Check sheet for the modelled part. Datum: model origin and axes. Units: mm. A direction names the side the tool comes from. Give positions to 0.01 mm unless a question says otherwise; leave off trailing zeros. Order: outer loops, then holes, each group sorted by start corner. A loop starts at its lowest first (then second) coordinate and runs counter-clockwise, first axis right, second up.
from build123d import *

# Parameters (mm, degrees)
SKETCH1_W           = 12.7
SKETCH1_H           = 5.08
BOSS_EXTRUDE1_DEPTH = 63.5
SKETCH2_W           = 5.334
SKETCH2_H           = 30.734
CUT_EXTRUDE1_DEPTH  = 3.175


with BuildPart() as part:
    # Sketch1 → Boss-Extrude1 (new body)
    with BuildSketch(Plane.XY):
        Rectangle(SKETCH1_W, SKETCH1_H)
        with BuildLine():
            Line((-73.690101608, 45.085), (-78.089510659, 42.545))
            ThreePointArc((-78.089510659, 42.545), (0, -2.54), (78.089510659, 42.545))
            Line((78.089510659, 42.545), (73.690101608, 45.085))
            ThreePointArc((73.690101608, 45.085), (0, 2.54), (-73.690101608, 45.085))
        make_face()
    extrude(amount=BOSS_EXTRUDE1_DEPTH)

    # Sketch2 → Cut-Extrude1 (cut)
    with BuildSketch(Plane.XZ.offset(2.54)):
        with Locations((0.1143, 40.64)):
            Rectangle(SKETCH2_W, SKETCH2_H)
    extrude(amount=-CUT_EXTRUDE1_DEPTH, mode=Mode.SUBTRACT)


solid = part.part
1) Section check B-B, the plane z = 29. Record the cut outline in (x, y) (3 decimals).
Recorded:
outline: (-78.09, 42.545) arc R90.17 ccw to (-6.35, -2.316) - (-6.35, -2.54) - (-2.553, -2.54) - (-2.553, 0.635) - (2.781, 0.635) - (2.781, -2.54) - (6.35, -2.54) - (6.35, -2.316) arc R90.17 ccw to (78.09, 42.545) - (73.69, 45.085) arc R85.09 cw to (-73.69, 45.085) - close
2) Section check D-D, the plane z = 17.5. Record the cut outline in (x, y) (3 decimals).
Recorded:
outline: (-78.09, 42.545) arc R90.17 ccw to (-6.35, -2.316) - (-6.35, -2.54) - (6.35, -2.54) - (6.35, -2.316) arc R90.17 ccw to (78.09, 42.545) - (73.69, 45.085) arc R85.09 cw to (-73.69, 45.085) - close
3) Section check C-C, the plane y = 31.5. Record the cut outline in (x, z).
Recorded:
outline: (-70.57, 0) - (-63.95, 0) - (-63.95, 63.5) - (-70.57, 63.5) - close; (63.95, 0) - (70.57, 0) - (70.57, 63.5) - (63.95, 63.5) - close
4) Section check A-A, the plane y = 40.5. Record the cut outline in (x, z).
Recorded:
outline: (-76.87, 0) - (-70.85, 0) - (-70.85, 63.5) - (-76.87, 63.5) - close; (70.85, 0) - (76.87, 0) - (76.87, 63.5) - (70.85, 63.5) - close
5) Depth check by flat-ended pin: pin 1 Ø4 at (x, z) = (29.5, 34) entering from +Y; pin 2 Ø1.5 at (y, z) = (24.5, 41.5) entering from +X; pin 3 Ø3 at (y, z) = (9, 52) entering from +X. Enter the tip coordinate at first touch or a pass-through.
Recorded:
pin 1: stops at y = 8.59
pin 2: stops at x = 65.11
pin 3: stops at x = 46.71
6) Set-up check for faces 1 (the face through (-75.86, 43.83, 31.31)), 2 (the face through (0, -1, 56.007)): record each of +Z, -Z, +X, -X, +Y, -Y from which the full face is reachable in a straight line by a thin tool's end or side.
Recorded:
face 1: +Z, -Z, -X, +Y
face 2: -Y
7) Material ranges on L1, parallel to X at y = 41, z = 50.5; L2, parallel to Y at x = 0.5, z = 31 (3 decimals); L3, parallel to X at y = 22, z = 19, recorded low to high.
Recorded:
L1: x = -77.18 to -71.18, 71.18 to 77.18
L2: y = 0.635 to 2.541
L3: x = -61.83 to -54.16, 54.16 to 61.83
